For this review, take the finished solid that the model builds, in its own axes (mm). Coordinates: 2 decimals unless noted, no trailing zeros. Loops run counter-clockwise (first coordinate to the right, second up) from the corner with the lowest first, then second, coordinate; pieces in that order, holes last. Notation, with made-up numbers: M -1,39.25 L 52,39.25 A16 cw 52,48.25 Z; hole C 4,-19.5 d2. An arc over 180 degrees is marked long. Write each question's results on one line, items separated by ' | '. Start each with the question number.
Autodesk Inventor part; units mm, degrees
ref_plane "YZ Plane" through (0, 0, 0) normal (1, 0, 0) x (0, 1, 0)
ref_plane "XZ Plane" through (0, 0, 0) normal (0, 1, 0) x (-1, 0, 0)
ref_plane "XY Plane" through (0, 0, 0) normal (0, 0, 1) x (1, 0, 0)
sketch "Sketch1" plane through (0, 0, 0) normal (0, 0, 1) x (1, 0, 0)
  circle A0 centre (134.3503, 224.3503) radius 2
  arc A1 (-3.5355, 93.5355) -> (-4.9889, 89.6672) centre (0, 90) ccw
  arc A2 (137.8858, 220.8148) -> (130.8148, 227.8858) centre (134.3503, 224.3503) ccw
  arc A3 (-1.9989, -0.0666) -> (1.9987, -0.0722) centre (0, 0) ccw
  circle A4 centre (56.5685, 146.5685) radius 2
  line L0 (-5, 90) -> (-1.9989, -0.0666)
  line L1 (130.8148, 227.8858) -> (-3.5355, 93.5355)
  line L2 (137.8858, 220.8148) -> (5.1833, 88.1122)
  line L3 (5.1833, 88.1122) -> (1.9987, -0.0722)
  dimension "d5" = 4
  dimension "d6" = 10
  dimension "d7" = 10
  dimension "d8" = 4
  dimension "d9" = 4
  dimension "d23" = 90
  dimension "d30" = 5
  dimension "d45" = 80
  dimension "d46" = 110
  dimension "d47" = 135
extrude "Extrusion2" add sketch "Sketch1" along normal blind 10 contours L1 A2 L2 L3 A3 L0 A1
fillet "Fillet1" radius 1 1 edges at (54.5685, 146.5685, 10)
fillet "Fillet2" radius 1 3 edges at (54.5685, 146.5685, 0) (132.3503, 224.3503, 0) (132.3503, 224.3503, 10)
equation "\"BendRadius\" = Thickness"
equation "\"BendReliefWidth\" = Thickness"
equation "\"BendReliefDepth\" = 0.5 * Thickness"
equation "\"CornerReliefSize\" = 4 * Thickness"
equation "\"MinimumRemnant\" = 2 * Thickness"
equation "\"TransitionRadius\" = BendRadius"
equation "\"JacobiRadiusSize\" = Thickness"
equation "\"GapSize\" = Thickness"
properties part number "Leg Spider Crab" material "Aluminum 6061"
Q1. Take a section at A-A, the plane z = 5.25. Give the boundary of the cut face in (x, y), then the cut area to 3 significant figures.
Q2. Take a section at B-B, the plane y = 54.5. Give the boundary of the cut face in (x, z).
Q3. Take a section at C-C, the plane x = 117. Give the boundary of the cut face in (y, z).
Q4. Insertion check: P1, Ø2.5, axis at x = 134.35, y = 224.35, coming from the +Z side; P2, Ø1.5, axis at y = 75.5, z = 4, coming from the -X side; P3, Ø3, axis at x = 100, z = 8, coming from the +Y side; P4, Ø4, axis at x = 60.5, z = 5, coming from the -Y side. Each pin has a flat end and moves straight along its axis. Give the tip position at first contact, or say it passes through.
Q5. To check wall thickness, follow line 1 along Y through (x, z) = (56, 1.25); line 2 along X through (y, z) = (148, 8.5); line 3 along X through (y, z) = (87, 5). State the ranges of each line that lie inside material, in increasing order.
Results:
1) outline: M -5,90 L -2,-0.07 A2 ccw 2,-0.07 L 5.18,88.11 L 137.89,220.81 A5 ccw 130.81,227.89 L -3.54,93.54 A5 ccw Z; hole C 56.57,146.57 d4; hole C 134.35,224.35 d4 | area: 2,560 mm^2
2) outline: M -3.82,0 L 3.97,0 L 3.97,10 L -3.82,10 Z
3) outline: M 199.93,0 L 214.07,0 L 214.07,10 L 199.93,10 Z
4) P1: through | P2: x = -4.54 | P3: y = 198.57 | P4: y = 141.43
5) line 1: 138.93 to 144.65, 148.49 to 153.07 | line 2: 50.93 to 55.17, 57.97 to 65.07 | line 3: -4.9 to 5.14
